Read the model definition and answer for the solid it produces. Units are mm, in the model's axes. Coordinates: 2 decimals unless noted, no trailing zeros. Loops run counter-clockwise (first coordinate to the right, second up) from the corner with the lowest first, then second, coordinate; pieces in that order, holes last. Notation, with made-up numbers: (57.5, 47) -> (104.5, 47) arc R25 cw to (104.5, 69) -> close; hole circle Ø8 at (68, -11). An arc over 180 degrees is marked (long way). Answer as a JSON object with one key per item and string values. Group by question number.
1) Consider probe 1 along X at (y, z) = (4.65, 8); probe 2 along Y at (x, z) = (-0.5, 113.5); probe 3 along X at (y, z) = (0, 157). Determine where each line is inside the solid, lowest interval first. Write a range as [from, to].
2) Section A-A, the plane y = 0 is taken. Give the vertices of the cut face in (x, z).
3) Section B-B, the plane z = 232 is taken. Give the vertices of the cut face in (x, y).
4) Section D-D, the plane z = 200 is taken. Give the vertices of the cut face in (x, y), plus the area to 3 significant figures.
5) Section C-C, the plane x = 5 is taken. Give the vertices of the cut face in (y, z), plus the area to 3 significant figures.
6) Flat-ended cylindrical pins translate along their axes: P1, Ø5, axis at x = -5, z = 8, coming from the +Y side; P2, Ø3, axis at x = 0, z = 120, coming from the -Y side. Find the tip coordinate at first contact, or state that the pin passes through.
from build123d import *

# Parameters (mm, degrees)
SKETCH_1_W          = 20
SKETCH_1_H          = 10
SKETCH_1_W_2        = 17
SKETCH_1_H_2        = 7
EXTRUDE_1_DEPTH     = 240
SKETCH_2_R          = 2.15
SKETCH_2_R_2        = 2.5
CUT_EXTRUDE_1_DEPTH = 241.416305603
SKETCH_3_R          = 2.15
CUT_EXTRUDE_2_DEPTH = 241.883789409


with BuildPart() as part:
    # ｽｹｯﾁ1 → 押し出し-薄板1 (new body)
    with BuildSketch(Plane.XY):
        Rectangle(SKETCH_1_W, SKETCH_1_H)
        Rectangle(SKETCH_1_W_2, SKETCH_1_H_2, mode=Mode.SUBTRACT)
    extrude(amount=EXTRUDE_1_DEPTH)

    # ｽｹｯﾁ2 → ｶｯﾄ - 押し出し1 (cut, through all)
    with BuildSketch(Plane(origin=(0, 5, 0), x_dir=(1, 0, 0), z_dir=(0, 1, 0))):
        with Locations(Location((5, -232, 0), (0, 0, 270))):
            Circle(SKETCH_2_R)
        with Locations(Location((-5, -232, 0), (0, 0, 270))):
            Circle(SKETCH_2_R)
        with Locations(Location((5, -8, 0), (0, 0, 270))):
            Circle(SKETCH_2_R)
        with Locations(Location((-5, -8, 0), (0, 0, 270))):
            Circle(SKETCH_2_R)
        with Locations(Location((0, -40, 0), (0, 0, 270))):
            Circle(SKETCH_2_R_2)
        with Locations(Location((0, -200, 0), (0, 0, 270))):
            Circle(SKETCH_2_R_2)
        with Locations(Location((0, -120, 0), (0, 0, 270))):
            Circle(SKETCH_2_R_2)
    extrude(amount=-CUT_EXTRUDE_1_DEPTH, mode=Mode.SUBTRACT)

    # ｽｹｯﾁ3 → ｶｯﾄ - 押し出し2 (cut, through all)
    with BuildSketch(Plane(origin=(10, 0, 0), x_dir=(0, 0, -1), z_dir=(1, 0, 0))):
        with Locations((-105, 0)):
            Circle(SKETCH_3_R)
        with Locations(Location((-135, 0, 0), (0, 0, 90))):
            Circle(SKETCH_3_R)
    extrude(amount=-CUT_EXTRUDE_2_DEPTH, mode=Mode.SUBTRACT)


solid = part.part
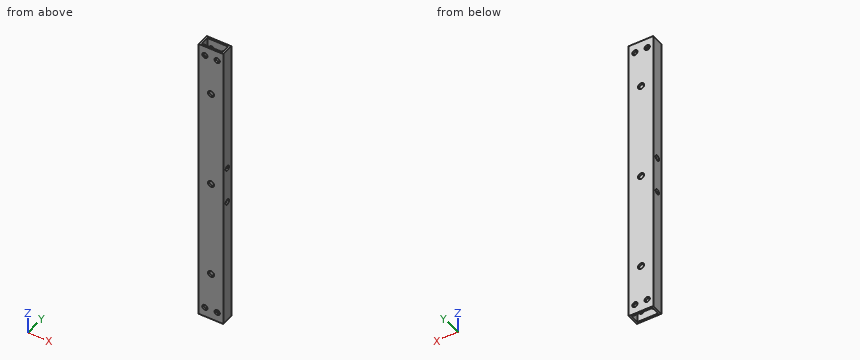
Determined:
{
 "1": {"probe 1": "[-10, -7.15], [-2.85, 2.85], [7.15, 10]", "probe 2": "[-5, -3.5], [3.5, 5]", "probe 3": "[-10, -8.5], [8.5, 10]"},
 "2": {"outline": "(-10, 0) -> (-8.5, 0) -> (-8.5, 102.85) -> (-10, 102.85) -> close; (-10, 107.15) -> (-8.5, 107.15) -> (-8.5, 132.85) -> (-10, 132.85) -> close; (-10, 137.15) -> (-8.5, 137.15) -> (-8.5, 240) -> (-10, 240) -> close; (8.5, 0) -> (10, 0) -> (10, 102.85) -> (8.5, 102.85) -> close; (8.5, 107.15) -> (10, 107.15) -> (10, 132.85) -> (8.5, 132.85) -> close; (8.5, 137.15) -> (10, 137.15) -> (10, 240) -> (8.5, 240) -> close"},
 "3": {"outline": "(-10, -5) -> (-7.15, -5) -> (-7.15, -3.5) -> (-8.5, -3.5) -> (-8.5, 3.5) -> (-7.15, 3.5) -> (-7.15, 5) -> (-10, 5) -> close; (-2.85, -5) -> (2.85, -5) -> (2.85, -3.5) -> (-2.85, -3.5) -> close; (-2.85, 3.5) -> (2.85, 3.5) -> (2.85, 5) -> (-2.85, 5) -> close; (7.15, -5) -> (10, -5) -> (10, 5) -> (7.15, 5) -> (7.15, 3.5) -> (8.5, 3.5) -> (8.5, -3.5) -> (7.15, -3.5) -> close"},
 "4": {"outline": "(-10, -5) -> (-2.5, -5) -> (-2.5, -3.5) -> (-8.5, -3.5) -> (-8.5, 3.5) -> (-2.5, 3.5) -> (-2.5, 5) -> (-10, 5) -> close; (2.5, -5) -> (10, -5) -> (10, 5) -> (2.5, 5) -> (2.5, 3.5) -> (8.5, 3.5) -> (8.5, -3.5) -> (2.5, -3.5) -> close", "area": "66.0 mm²"},
 "5": {"outline": "(-5, 0) -> (-3.5, 0) -> (-3.5, 5.85) -> (-5, 5.85) -> close; (-5, 10.15) -> (-3.5, 10.15) -> (-3.5, 229.85) -> (-5, 229.85) -> close; (-5, 234.15) -> (-3.5, 234.15) -> (-3.5, 240) -> (-5, 240) -> close; (3.5, 0) -> (5, 0) -> (5, 5.85) -> (3.5, 5.85) -> close; (3.5, 10.15) -> (5, 10.15) -> (5, 229.85) -> (3.5, 229.85) -> close; (3.5, 234.15) -> (5, 234.15) -> (5, 240) -> (3.5, 240) -> close", "area": "694 mm²"},
 "6": {"P1": "y = 5", "P2": "through"}
}
